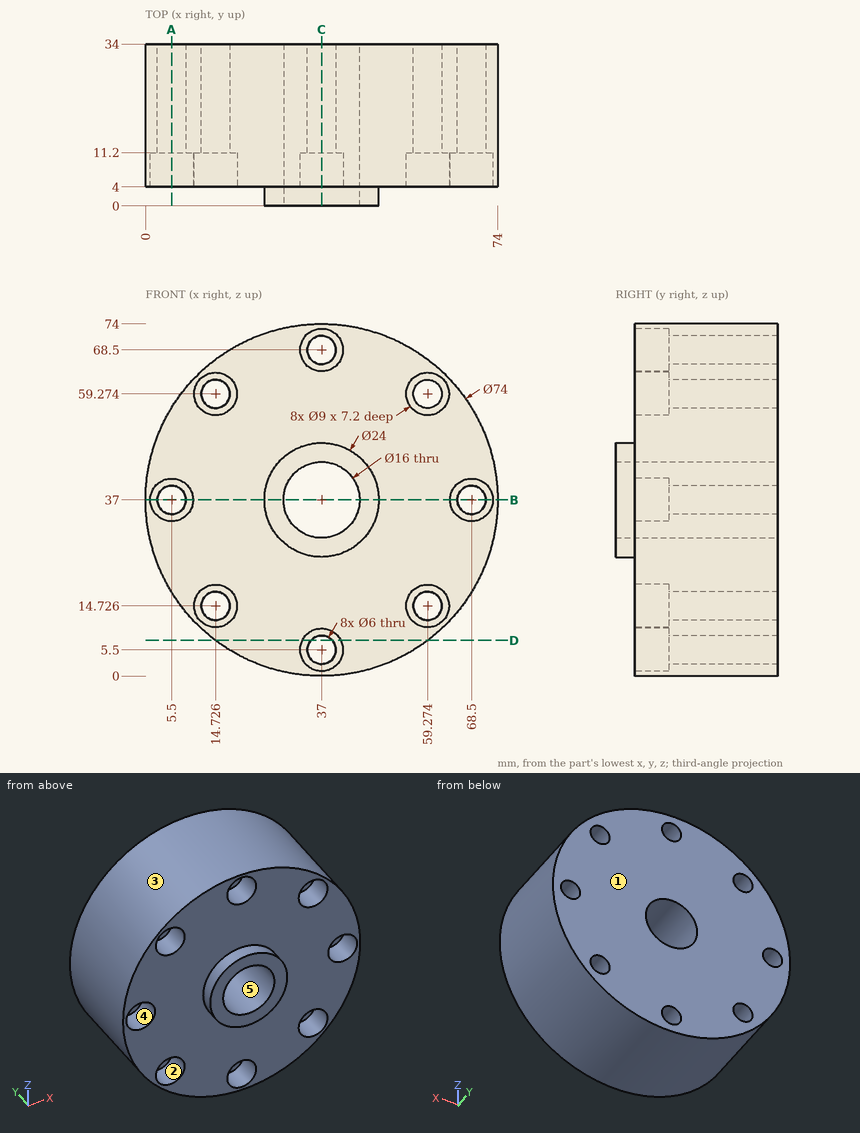
Print and shaded views of the part. All mm, measured from the part's lowest x, y and z. A direction names the side the tool comes from. Give positions to 0.01 mm unless a question says otherwise; leave off trailing zeros. Order: outer loops, then holes, each group sorted by start corner. A loop starts at its lowest first (then second) coordinate and runs counter-clockwise, first axis right, second up. Notation, with made-up numbers: (29.25, 38) - (35.25, 38) arc R12 cw to (35.25, 47) - close; hole circle Ø10 at (73.5, 53.5). An arc over 180 degrees is marked (long way). One line per item, written item: value.
Item 1: Two-plate mould, pull along Z, no slides. Class the marked faces 1, 2 and 3: released by +Z, released by -Z, zero draft, split by the parting line, or undercut.
Response values:
face 1: zero draft
face 2: undercut
face 3: split by the parting line
Item 2: Tool access for the marked faces 4 and 5: list every direction of +Z, -Z, +X, -X, +Y, -Y with a clear straight run to the whole face (end or side of a thin tool).
Response values:
face 4: -Y
face 5: +Y, -Y
Item 3: Slice it at D-D (z = 7.5). List the corners of the cut face in (x, y).
Response values:
outline: (14.67, 4) - (32.97, 4) - (32.97, 11.2) - (34.76, 11.2) - (34.76, 34) - (14.67, 34) - close; (39.24, 11.2) - (41.03, 11.2) - (41.03, 4) - (59.33, 4) - (59.33, 34) - (39.24, 34) - close
Item 4: Slice it at A-A (x = 5.5). List the corners of the cut face in (y, z).
Response values:
outline: (4, 17.59) - (34, 17.59) - (34, 34) - (11.2, 34) - (11.2, 32.5) - (4, 32.5) - close; (4, 41.5) - (11.2, 41.5) - (11.2, 40) - (34, 40) - (34, 56.41) - (4, 56.41) - close
Item 5: Pin check, flat tips, straight feed: pin 1 Ø6 at (x, y) = (29, 23.5) entering from -Z; pin 2 Ø8 at (x, z) = (37, 68.5) entering from -Y; pin 3 Ø3 at (y, z) = (21, 34) entering from +X; pin 4 Ø9.5 at (x, z) = (5.5, 37) entering from +Y. Stop position of each tip, or through.
Response values:
pin 1: z = 0.34
pin 2: y = 11.2
pin 3: x = 73.97
pin 4: y = 34
Item 6: Slice it at C-C (x = 37). List the corners of the cut face in (y, z), then the cut area to 3 significant figures.
Response values:
outline: (0, 25) - (4, 25) - (4, 10) - (11.2, 10) - (11.2, 8.5) - (34, 8.5) - (34, 29) - (0, 29) - close; (0, 45) - (34, 45) - (34, 65.5) - (11.2, 65.5) - (11.2, 64) - (4, 64) - (4, 49) - (0, 49) - close; (4, 0) - (34, 0) - (34, 2.5) - (11.2, 2.5) - (11.2, 1) - (4, 1) - close; (4, 73) - (11.2, 73) - (11.2, 71.5) - (34, 71.5) - (34, 74) - (4, 74) - close
area: 1,370 mm2
Item 7: Wall check: line 1 (Z direction, x = 58, y = 17.5); line 2 (Y direction, x = 30, z = 7.5); line 3 (Z direction, x = 34.5, y = 31) (1 decimal). Give the ranges that are in metal, low to high.
Response values:
line 1: 6.54 to 12.01, 17.44 to 56.56, 61.99 to 67.46
line 2: 4 to 34
line 3: 0.1 to 3.8, 7.2 to 29.4, 44.6 to 66.8, 70.2 to 73.9
Item 8: Slice it at B-B (z = 37). List the corners of the cut face in (x, y), then the cut area to 3 significant figures.
Response values:
outline: (0, 4) - (1, 4) - (1, 11.2) - (2.5, 11.2) - (2.5, 34) - (0, 34) - close; (8.5, 11.2) - (10, 11.2) - (10, 4) - (25, 4) - (25, 0) - (29, 0) - (29, 34) - (8.5, 34) - close; (45, 0) - (49, 0) - (49, 4) - (64, 4) - (64, 11.2) - (65.5, 11.2) - (65.5, 34) - (45, 34) - close; (71.5, 11.2) - (73, 11.2) - (73, 4) - (74, 4) - (74, 34) - (71.5, 34) - close
area: 1,370 mm2
